from build123d import *

# Parameters (mm, degrees)
BOSS_EXTRUDE1_DEPTH = 4
BOSS_EXTRUDE2_DEPTH = 4
SKETCH3_R           = 1.25
BOSS_EXTRUDE3_DEPTH = 16
FILLET1_R           = 1
FILLET2_R           = 0.5
FILLET3_R           = 0.75


with BuildPart() as part:
    # Sketch1 → Boss-Extrude1 (new body)
    with BuildSketch(Plane.XY):
        Polygon((2.3, -4.75), (3.5, -4.75), (3.5, 4.75), (2.3, 4.75), (2.3, 2.65), (-0.2, 2.65), (-0.2, 4.75), (-3.5, 4.75), (-3.5, -4.75), (-0.2, -4.75), (-0.2, -2.65), (2.3, -2.65), align=None)
    extrude(amount=BOSS_EXTRUDE1_DEPTH)

    # Sketch2 → Boss-Extrude2 (add)
    with BuildSketch(Plane(origin=(0, 0, 0), x_dir=(-1, 0, 0), z_dir=(0, 0, -1))):
        Polygon((-6, 1.5), (-6, -1), (-3.5, -4.75), (-3.5, 4.75), align=None)
    extrude(amount=-BOSS_EXTRUDE2_DEPTH)

    # Sketch3 → Boss-Extrude3 (add)
    with BuildSketch(Plane.XY.offset(4)):
        with Locations((-1.5, 0)):
            Circle(SKETCH3_R)
    extrude(amount=BOSS_EXTRUDE3_DEPTH)

    # Fillet1
    fillet1_edges = [part.edges().sort_by_distance(p)[0] for p in [
        (-3.5, -4.75, 2),
        (-3.5, 4.75, 2),
        (3.5, 4.75, 2),
        (3.5, -4.75, 2),
        (6, -1, 2),
        (6, 1.5, 2),
    ]]
    fillet(fillet1_edges, radius=FILLET1_R)

    # Fillet2
    fillet2_edges = [part.edges().sort_by_distance(p)[0] for p in [
        (-2.75, 0, 4),
    ]]
    fillet(fillet2_edges, radius=FILLET2_R)

    # Fillet3
    fillet3_edges = [part.edges().sort_by_distance(p)[0] for p in [
        (-2.75, 0, 20),
    ]]
    fillet(fillet3_edges, radius=FILLET3_R)


solid = part.part
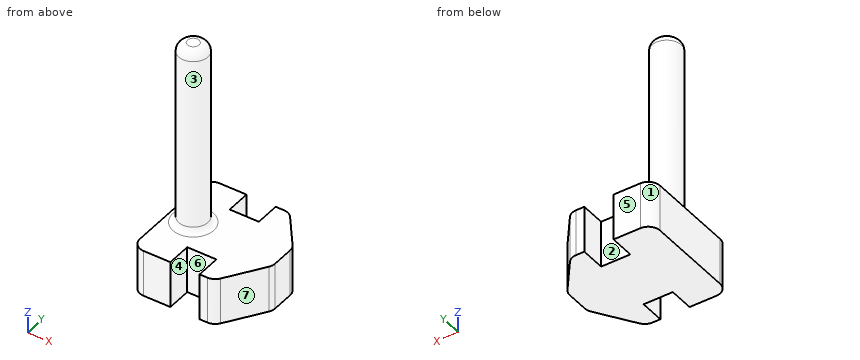
Check sheet for the modelled part. Datum: model origin and axes. Units: mm. Face numbers are marked on the shaded views. A direction names the side the tool comes from. Give positions to 0.01 mm unless a question says otherwise; leave off trailing zeros. Write each loop counter-clockwise with the first axis right and the second up, starting at its lowest first coordinate (ties: lowest second). Pieces come first, ordered by that corner, then holes. Notation, with made-up numbers: (89, 37) -> (127, 37) arc R23 cw to (127, 57) -> close; hole circle Ø10 at (72.5, 6.5). An arc over 180 degrees is marked (long way). Write item = value, one per line.
Item 1: Sectioned sample at A-A on y = -4. Record the boundary of the cut face in (x, z), and give its area (3 significant figures).
Output:
outline = (-3.47, 0) -> (-0.2, 0) -> (-0.2, 4) -> (-3.47, 4) -> close; (2.3, 0) -> (4, 0) -> (4, 4) -> (2.3, 4) -> close
area = 19.9 mm^2
Item 2: Release check for a two-part mould opening along X. For the marked faces 5, 6 and 7 record: +X half, -X half, draft (parallel to the pull), parting line (faces both ways), or undercut.
Output:
face_5 = draft
face_6 = undercut
face_7 = +X half
Item 3: Tool access check on the marked faces 1, 2, 3 and 4. Record the directions out of +Z, -Z, +X, -X, +Y, -Y that give a thin tool (end or side, any length) a straight path to the whole face; none if there is none.
Output:
face_1 = +Z, -Z, -X, +Y
face_2 = +Z, -Z, +Y
face_3 = +Z
face_4 = +Z, -Z, -Y
Item 4: Sectioned sample at C-C on x = 4.5. Record the boundary of the cut face in (y, z).
Output:
outline = (-3.25, 0) -> (3.45, 0) -> (3.45, 4) -> (-3.25, 4) -> close
Item 5: Sectioned sample at B-B on x = 1.75. Record the boundary of the cut face in (y, z), and give its area (3 significant figures).
Output:
outline = (-2.65, 0) -> (2.65, 0) -> (2.65, 4) -> (-2.65, 4) -> close
area = 21.2 mm^2
Item 6: Gauge pin test, flat ends, axial feed: pin 1 (3 mm diameter, centred on y = -3, z = 3.5, fed in from +X); pin 2 (5 mm diameter, centred on y = -1.5, z = 14.5, fed in from +X); pin 3 (1.7 mm diameter, centred on y = -3.5, z = 2, fed in from +X); pin 4 (1.5 mm diameter, centred on y = 3, z = 15, fed in from -X). Record the tip position at first contact, or that the pin passes through.
Output:
pin_1 = 5.67
pin_2 = -0.25
pin_3 = 4.9
pin_4 = through
Item 7: Scan lines: probe 1 along Z at (x, y) = (-2, -3); probe 2 along Y at (x, z) = (-1.5, 10.5); probe 3 along X at (y, z) = (-3.5, 1.5). Record each from-to range of solid material in increasing order. Write a range as from..to.
Output:
probe_1 = 0..4
probe_2 = -1.25..1.25
probe_3 = -3.5..-0.2, 2.3..4.33
